Can you work these out from the model? Positions are in its coordinate system, mm. Face numbers are marked on the shaded views. A direction names the side the tool comes from. Give positions to 0.01 mm unless a question says otherwise; leave off trailing zeros. Loops run counter-clockwise (first coordinate to the right, second up) from the corner with the lowest first, then second, coordinate; pieces in that order, holes last. Notation, with made-up numbers: M 86,39 L 108,39 A22 cw 108,59 Z; hole C -28.5,-36 d1. An arc over 180 degrees is marked long. Put each result on its own line as item: value. Start each with the question number.
1) For the marked faces 4, 5 and 6, which set-ups out of +Z, -Z, +X, -X, +Y, -Y let a thin tool reach every point of the face, with its end or its side?
2) Please list where these lines run through material, in increasing order: line 1 along Y through (x, z) = (34, 30.5); line 2 along Y through (x, z) = (162, 48); line 3 along X through (y, z) = (16.5, 26.5). Write a range as from..to.
3) Imagine slicing it at D-D (x = 58.5). Write out the boundary of the cut face in (y, z), then the cut area to 3 significant figures.
4) For P1, Ø3, axis at x = 155.5, z = 23.5, coming from the +Y side; P2, Ø9.5, axis at y = 14.5, z = 37, coming from the -X side; P3, Ø1.5, axis at y = 13, z = 35.5, coming from the +X side, each with a flat end and sliding along its axis, tell me the tip position at first contact or that it passes through.
5) Imagine slicing it at B-B (z = 45). Write out the boundary of the cut face in (x, y), then the cut area to 3 significant figures.
6) If we mould it in two halves opening along X, with no side actions, what happens to the marked faces 1, 2 and 3? For each: +X half, -X half, draft (parallel to the pull), parting line (faces both ways), or undercut.
7) Imagine slicing it at C-C (y = 12). Write out the boundary of the cut face in (x, z), then the cut area to 4 significant figures.
8) Imagine slicing it at A-A (x = 38). Write out the boundary of the cut face in (y, z), then the cut area to 3 significant figures.
from build123d import *

# Parameters (mm, degrees)
BOSS_EXTRUDE1_DEPTH = 50


with BuildPart() as part:
    # Sketch1 → Boss-Extrude1 (new body)
    with BuildSketch(Plane.XY):
        with BuildLine():
            Line((0, 0), (0, 4))
            Line((0, 4), (57, 4))
            ThreePointArc((57, 4), (59.121320344, 4.878679656), (60, 7))
            Line((60, 7), (60, 18.840970938))
            ThreePointArc((60, 18.840970938), (58.965605224, 21.107332803), (56.575735931, 21.810819419))
            Line((56.575735931, 21.810819419), (46.211060633, 20.330151519))
            ThreePointArc((46.211060633, 20.330151519), (45.999463625, 20.307547374), (45.786796564, 20.3))
            Line((45.786796564, 20.3), (0, 20.3))
            Line((0, 20.3), (0, 30.3))
            Line((0, 30.3), (70, 30.3))
            Line((70, 30.3), (94.3, 6))
            Line((94.3, 6), (174.3, 6))
            Line((174.3, 6), (174.3, 0))
            Line((174.3, 0), (0, 0))
        make_face()
    extrude(amount=BOSS_EXTRUDE1_DEPTH)


solid = part.part
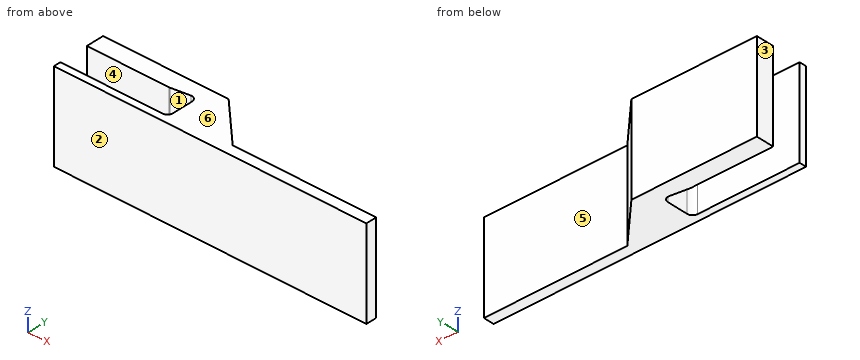
Recorded:
1. face 4: +Z, -Z, -X
1. face 5: +Z, -Z, +X, +Y
1. face 6: +Z, +X, -X, +Y, -Y
2. line 1: 0..4, 20.3..30.3
2. line 2: 0..6
2. line 3: 60..83.8
3. outline: M 0,0 L 4.4,0 L 4.4,50 L 0,50 Z; M 21.44,0 L 30.3,0 L 30.3,50 L 21.44,50 Z
3. area: 663 mm²
4. P1: y = 6
4. P2: x = 59.97
4. P3: x = 88.05
5. outline: M 0,0 L 174.3,0 L 174.3,6 L 94.3,6 L 70,30.3 L 0,30.3 L 0,20.3 L 45.79,20.3 A3 ccw 46.21,20.33 L 56.58,21.81 A3 cw 60,18.84 L 60,7 A3 cw 57,4 L 0,4 Z
5. area: 2,050 mm²
6. face 1: undercut
6. face 2: draft
6. face 3: -X half
7. outline: M 60,0 L 88.3,0 L 88.3,50 L 60,50 Z
7. area: 1,415 mm²
8. outline: M 0,0 L 4,0 L 4,50 L 0,50 Z; M 20.3,0 L 30.3,0 L 30.3,50 L 20.3,50 Z
8. area: 700 mm²
